Design review of the part built by this model. Coordinates are the model's own, in mm. A direction names the side the tool comes from. Give positions to 0.01 mm unless a question says otherwise; leave off trailing zeros. Order: outer loops, then holes, each group sorted by start corner. A loop starts at its lowest first (then second) coordinate and runs counter-clockwise, first axis right, second up. Notation, with made-up numbers: (74.25, 52.25) -> (78.25, 52.25) arc R13 ccw to (78.25, 66.25) -> close; hole circle Ø6 at (40.25, -7). An arc over 180 degrees is marked (long way). Return JSON: item names as keys, results as strings.
```python
from build123d import *

# Parameters (mm, degrees)
EXTRUDE_1_DEPTH     = 82
CUT_EXTRUDE_1_REACH = 109.835
SKETCH_2_R          = 1.6
SKETCH_3_R          = 1.6
EXTRUDE_2_DEPTH     = 10
CUT_EXTRUDE_2_DEPTH = 10
SKETCH_5_R          = 3
CUT_EXTRUDE_3_DEPTH = 10
EXTRUDE_START       = -10
SKETCH_6_R          = 1.6
EXTRUDE_3_DEPTH     = 10
CUT_EXTRUDE_4_REACH = 114.322
CUT_EXTRUDE_START   = -10
SKETCH_8_R          = 3
CUT_EXTRUDE_5_DEPTH = 10
FILLET_1_R          = 4


with BuildPart() as part:
    # 草图1 → 凸台-拉伸1 (new body)
    with BuildSketch(Plane.XY):
        Polygon((-31.5, 18.115697408), (28.5, -16.525318744), (28.5, -33.884302592), (31.5, -33.884302592), (31.5, -14.793267936), (28.5, -13.061217128), (-28.5, 19.847748215), (-28.5, 36.115697408), (-31.5, 36.115697408), align=None)
    extrude(amount=EXTRUDE_1_DEPTH)

    # 草图2 → 切除-拉伸1 (cut, up to next)
    with BuildSketch(Plane(origin=(-28.5, 0, 0), x_dir=(0, 0, -1), z_dir=(1, 0, 0)), mode=Mode.PRIVATE) as cut_extrude_1_sk1:
        with Locations(Location((-67, 31.115697408, 0), (0, 0, 90))):
            Circle(SKETCH_2_R)
    cut_extrude_1_tool1 = extrude(cut_extrude_1_sk1.sketch, amount=-CUT_EXTRUDE_1_REACH, mode=Mode.PRIVATE) & part.part
    # 草图2 → 切除-拉伸1 (cut, up to next)
    with BuildSketch(Plane(origin=(-28.5, 0, 0), x_dir=(0, 0, -1), z_dir=(1, 0, 0)), mode=Mode.PRIVATE) as cut_extrude_1_sk2:
        with Locations(Location((-15, 31.115697408, 0), (0, 0, 90))):
            Circle(SKETCH_2_R)
    cut_extrude_1_tool2 = extrude(cut_extrude_1_sk2.sketch, amount=-CUT_EXTRUDE_1_REACH, mode=Mode.PRIVATE) & part.part
    add(cut_extrude_1_tool1.solids().sort_by_distance((-28.5, 31.115697, 67))[0], mode=Mode.SUBTRACT)
    add(cut_extrude_1_tool2.solids().sort_by_distance((-28.5, 31.115697, 15))[0], mode=Mode.SUBTRACT)

    # 草图3 → 凸台-拉伸2 (add)
    with BuildSketch(Plane(origin=(0, 0, 0), x_dir=(-1, 0, 0), z_dir=(0, 0, -1))):
        with BuildLine():
            Line((-28.5, -33.884302592), (-23.5, -33.884302592))
            ThreePointArc((-23.5, -33.884302592), (-18.5, -28.884302592), (-23.5, -23.884302592))
            Line((-23.5, -23.884302592), (-28.5, -23.884302592))
            Line((-28.5, -23.884302592), (-28.5, -33.884302592))
        make_face()
        with Locations((-23.5, -28.884302592)):
            Circle(SKETCH_3_R, mode=Mode.SUBTRACT)
    extrude(amount=-EXTRUDE_2_DEPTH)

    # 草图4 → 切除-拉伸2 (cut)
    with BuildSketch(Plane.XZ.offset(33.884302592)):
        with BuildLine():
            Line((15.48929146, 10), (15.48929146, 5))
            Line((15.48929146, 5), (18.5, 5))
            add(Edge.make_bspline(
                [(28.5, 10), (26.534032888, 6.656358998), (22.320432112, 5.379510278), (18.5, 5)],
                knots=[0, 0, 0, 0, 1, 1, 1, 1], degree=3))
            Line((28.5, 10), (15.48929146, 10))
        make_face()
    extrude(amount=-CUT_EXTRUDE_2_DEPTH, mode=Mode.SUBTRACT)

    # 草图5 → 切除-拉伸3 (cut)
    with BuildSketch(Plane(origin=(0, 0, 5), x_dir=(-1, 0, 0), z_dir=(0, 0, -1))):
        with Locations((-23.5, -28.884302592)):
            Circle(SKETCH_5_R)
    extrude(amount=-CUT_EXTRUDE_3_DEPTH, mode=Mode.SUBTRACT)

    # 草图6 → 凸台-拉伸3 (add)
    with BuildSketch(Plane.XY.offset(82).offset(EXTRUDE_START)):
        with BuildLine():
            Line((28.5, -23.884302592), (23.5, -23.884302592))
            ThreePointArc((23.5, -23.884302592), (18.5, -28.884302592), (23.5, -33.884302592))
            Line((23.5, -33.884302592), (28.5, -33.884302592))
            Line((28.5, -33.884302592), (28.5, -23.884302592))
        make_face()
        with Locations(Location((23.5, -28.884302592, 0), (0, 0, 180))):
            Circle(SKETCH_6_R, mode=Mode.SUBTRACT)
    extrude(amount=EXTRUDE_3_DEPTH)

    # 草图7 → 切除-拉伸4 (cut, up to next)
    with BuildSketch(Plane.XZ.offset(33.884302592), mode=Mode.PRIVATE) as cut_extrude_4_sk1:
        with BuildLine():
            Line((28.5, 72), (15.711275948, 72))
            Line((15.711275948, 72), (15.711275948, 77))
            Line((15.711275948, 77), (18.5, 77))
            add(Edge.make_bspline(
                [(28.5, 72), (25.18574882, 75.388408821), (22.578679104, 76.660150146), (18.5, 77)],
                knots=[0, 0, 0, 0, 1, 1, 1, 1], degree=3))
        make_face()
    cut_extrude_4_tool1 = extrude(cut_extrude_4_sk1.sketch, amount=-CUT_EXTRUDE_4_REACH, mode=Mode.PRIVATE) & part.part
    add(cut_extrude_4_tool1.solids().sort_by_distance((20.757737, -33.884303, 74.139279))[0], mode=Mode.SUBTRACT)

    # 草图8 → 切除-拉伸5 (cut)
    with BuildSketch(Plane.XY.offset(77).offset(CUT_EXTRUDE_START)):
        with Locations(Location((23.5, -28.884302592, 0), (0, 0, 180))):
            Circle(SKETCH_8_R)
    extrude(amount=CUT_EXTRUDE_5_DEPTH, mode=Mode.SUBTRACT)

    # 圆角1
    fillet_1_edges = [part.edges().sort_by_distance(p)[0] for p in [
        (28.5, -16.525318744, 41),
        (31.5, -14.793267936, 41),
        (-28.5, 19.847748215, 41),
        (28.5, -23.884302592, 77),
        (28.5, -23.884302592, 5),
    ]]
    fillet(fillet_1_edges, radius=FILLET_1_R)


solid = part.part
```
Item 1: Mouldability with a two-part tool opening along Z and no side actions: class faces 1 (the face through (-30, 36.116, 40)), 2 (the face through (7.1, -3.9, 0)), 3 (the face through (22, -30, 5)) as released by +Z, released by -Z, zero draft, split by the parting line, or undercut.
Result set:
{"face 1": "zero draft", "face 2": "released by -Z", "face 3": "undercut"}
Item 2: Machinability: for faces 4 (the face through (27.3, -22.74, 77.07)), 5 (the face through (22.2, -27.6, 77)), 6 (the face through (-28.5, 29, 40)), which of the approach directions +Z, -Z, +X, -X, +Y, -Y give a long, thin tool a straight path to every point of the face, cutting with its end or side? Answer none if there is none.
Result set:
{"face 4": "+Z, -Z, -X", "face 5": "none", "face 6": "+Z, -Z, +X, +Y"}
Item 3: Add section C-C (y = 26.5). Give the boundary of the cut face in (x, z), plus the area to 3 significant figures.
Result set:
{"outline": "(-31.5, 0) -> (-28.5, 0) -> (-28.5, 82) -> (-31.5, 82) -> close", "area": "246 mm^2"}
Item 4: For pin 1 (1 mm diameter, centred on y = -18.5, z = 50.5, fed in from -X); pin 2 (5 mm diameter, centred on y = 31.12, z = 15, fed in from -X); pin 3 (1 mm diameter, centred on x = -22, z = 44.5, fed in from -Y); pin 4 (4.5 mm diameter, centred on y = -25, z = 45, fed in from -X), all flat-tipped, find the tip position at first contact; note any pin that passes through.
Result set:
{"pin 1": "stops at x = 28.41", "pin 2": "stops at x = -31.5", "pin 3": "stops at y = 12.34", "pin 4": "stops at x = 28.5"}
Item 5: Wall thickness on L1, parallel to Y at x = -30, z = 67; L2, parallel to Y at x = -30.65, z = 67; L3, parallel to X at y = 18, z = 14.5: over which ranges is each line inside the solid? List them lowest first. Write a range as [from, to].
Result set:
{"L1": "y = [17.25, 29.52], [32.72, 36.12]", "L2": "y = [17.62, 29.52], [32.72, 36.12]", "L3": "x = [-31.3, -25.3]"}
Item 6: Add section A-A (z = 15). Give the boundary of the cut face in (x, y).
Result set:
{"outline": "(-31.5, 18.12) -> (26.5, -15.37) arc R4 cw to (28.5, -18.83) -> (28.5, -33.88) -> (31.5, -33.88) -> (31.5, -17.1) arc R4 ccw to (29.5, -13.64) -> (-26.5, 18.69) arc R4 cw to (-28.5, 22.16) -> (-28.5, 29.52) -> (-31.5, 29.52) -> close; (-31.5, 32.72) -> (-28.5, 32.72) -> (-28.5, 36.12) -> (-31.5, 36.12) -> close"}
Item 7: Add section B-B (z = 42). Give the boundary of the cut face in (x, y), plus the area to 3 significant figures.
Result set:
{"outline": "(-31.5, 18.12) -> (26.5, -15.37) arc R4 cw to (28.5, -18.83) -> (28.5, -33.88) -> (31.5, -33.88) -> (31.5, -17.1) arc R4 ccw to (29.5, -13.64) -> (-26.5, 18.69) arc R4 cw to (-28.5, 22.16) -> (-28.5, 36.12) -> (-31.5, 36.12) -> close", "area": "315 mm^2"}
Item 8: Add section D-D (x = 14). Give the boundary of the cut face in (y, z).
Result set:
{"outline": "(-8.15, 0) -> (-4.69, 0) -> (-4.69, 82) -> (-8.15, 82) -> close"}
